Work out the finished part from the listing and answer in its coordinate system (mm). Face numbers are marked on the shaded views. A direction names the side the tool comes from. Give positions to 0.01 mm unless a question says otherwise; leave off trailing zeros. Loops run counter-clockwise (first coordinate to the right, second up) from the corner with the lowest first, then second, coordinate; pieces in that order, holes last. Notation, with made-up numbers: M 55.25,63 L 89.25,63 A22 cw 89.25,86 Z; hole C -20,83 d4. An arc over 180 degrees is marked long. Write item = value, one per line. Start each with the question number.
1. Section C-C on z = 8 is taken. Determine the outline of the cut face in (x, y).
2. Section B-B on x = 0 is taken. Determine the outline of the cut face in (y, z).
3. Consider L1, parallel to X at y = 2, z = -1; L2, parallel to X at y = 6, z = 16.2; L3, parallel to Z at x = 5.75, y = 8. Determine where each line is inside the solid, lowest interval first. Write a range as [from, to].
4. For the marked faces 1 and 2, determine the directions among +Z, -Z, +X, -X, +Y, -Y from which every point of the face is accessible in a straight line to the end or side of a thin tool.
5. Flat-ended cylindrical pins translate along their axes: pin 1 Ø4 at (x, z) = (-4.5, 12) entering from -Y; pin 2 Ø1 at (x, z) = (-0.5, 7.5) entering from +Y; pin 3 Ø6 at (x, z) = (-5.5, -8.5) entering from +Y. Find the tip coordinate at first contact, or state that the pin passes through.
6. Section A-A on y = 6 is taken. Determine the outline of the cut face in (x, z).
7. The mould has two halves that part along X. Classify the marked faces 3, 4, 5 and 6: released by +X, released by -X, zero draft, split by the parting line, or undercut.
8. Section D-D on y = 1.75 is taken. Determine the outline of the cut face in (x, z).
```python
from build123d import *

# Parameters (mm, degrees)
SKETCH_1_W          = 17
SKETCH_1_H          = 33
EXTRUDE_1_DEPTH     = 10
CUT_EXTRUDE_START   = 1
SKETCH_2_W          = 15
SKETCH_2_H          = 32
CUT_EXTRUDE_1_DEPTH = 8
SKETCH_3_R          = 3
CUT_EXTRUDE_2_DEPTH = 22.083168642
CUT_EXTRUDE_START_2 = 9
SKETCH_5_W          = 17
SKETCH_5_H          = 32
CUT_EXTRUDE_3_DEPTH = 8
EXTRUDE_START       = 9
SKETCH_6_W          = 17
SKETCH_6_H          = 32
EXTRUDE_2_DEPTH     = 1
SKETCH_7_W          = 17
SKETCH_7_H          = 32
CUT_EXTRUDE_4_DEPTH = 1


with BuildPart() as part:
    # 스케치1 → 보스-돌출1 (new body)
    with BuildSketch(Plane(origin=(0, 0, 0), x_dir=(1, 0, 0), z_dir=(0, 1, 0))):
        Rectangle(SKETCH_1_W, SKETCH_1_H)
    extrude(amount=EXTRUDE_1_DEPTH)

    # 스케치2 → 컷-돌출1 (cut)
    with BuildSketch(Plane(origin=(0, 0, 0), x_dir=(1, 0, 0), z_dir=(0, 1, 0)).offset(CUT_EXTRUDE_START)):
        with Locations((0, 0.5)):
            Rectangle(SKETCH_2_W, SKETCH_2_H)
    extrude(amount=CUT_EXTRUDE_1_DEPTH, mode=Mode.SUBTRACT)

    # 스케치3 → 컷-돌출2 (cut, through all)
    with BuildSketch(Plane.XY):
        with Locations(Location((0, 6, 0), (0, 0, 90))):
            Circle(SKETCH_3_R)
    extrude(amount=CUT_EXTRUDE_2_DEPTH, mode=Mode.SUBTRACT)

    # 스케치5 → 컷-돌출3 (cut)
    with BuildSketch(Plane(origin=(0, 0, 0), x_dir=(1, 0, 0), z_dir=(0, 1, 0)).offset(CUT_EXTRUDE_START_2)):
        with Locations((0, 0.5)):
            Rectangle(SKETCH_5_W, SKETCH_5_H)
    extrude(amount=CUT_EXTRUDE_3_DEPTH, mode=Mode.SUBTRACT)


with BuildPart() as body_2:
    # 스케치6 → 보스-돌출2 (new body)
    with BuildSketch(Plane(origin=(0, 0, 0), x_dir=(1, 0, 0), z_dir=(0, 1, 0)).offset(EXTRUDE_START)):
        with Locations((0, 0.5)):
            Rectangle(SKETCH_6_W, SKETCH_6_H)
    extrude(amount=EXTRUDE_2_DEPTH)

    # 스케치7 → 컷-돌출4 (cut)
    with BuildSketch(Plane(origin=(0, 10, 0), x_dir=(1, 0, 0), z_dir=(0, 1, 0))):
        with Locations((0, 0.5)):
            Rectangle(SKETCH_7_W, SKETCH_7_H)
    extrude(amount=-CUT_EXTRUDE_4_DEPTH, mode=Mode.SUBTRACT)


solid = part.part
```
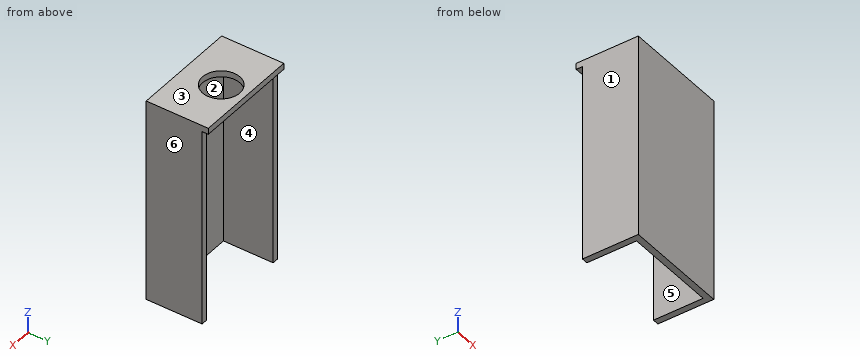
Verdict:
q1.outline = M -8.5,0 L 8.5,0 L 8.5,9 L 7.5,9 L 7.5,1 L -7.5,1 L -7.5,9 L -8.5,9 Z
q2.outline = M 0,-16.5 L 1,-16.5 L 1,15.5 L 3,15.5 L 3,16.5 L 0,16.5 Z; M 9,15.5 L 10,15.5 L 10,16.5 L 9,16.5 Z
q3.L1 = [-8.5, -7.5], [7.5, 8.5]
q3.L2 = [-8.5, -3], [3, 8.5]
q3.L3 = [15.5, 16.5]
q4.face_1 = +Z, -Z, -X, +Y, -Y
q4.face_2 = -Z, +Y
q5.pin_1 = 0
q5.pin_2 = 1
q5.pin_3 = 9
q6.outline = M -8.5,-16.5 L -7.5,-16.5 L -7.5,15.5 L -3,15.5 L -3,16.5 L -8.5,16.5 Z; M 3,15.5 L 7.5,15.5 L 7.5,-16.5 L 8.5,-16.5 L 8.5,16.5 L 3,16.5 Z
q7.face_3 = zero draft
q7.face_4 = undercut
q7.face_5 = undercut
q7.face_6 = released by +X
q8.outline = M -8.5,-16.5 L -7.5,-16.5 L -7.5,15.5 L 7.5,15.5 L 7.5,-16.5 L 8.5,-16.5 L 8.5,16.5 L -8.5,16.5 Z
